Geometry check sheet. Reference: drawing and pictorial views, mm from the part's lowest x, y, z. A direction names the side the tool comes from. Round coordinates to 2 decimals unless told otherwise and drop trailing zeros. Put each result on its own line as item: value. Start each with the question number.
(1) Material ranges on probe 1 along X at (y, z) = (1.25, 42.5); probe 2 along X at (y, z) = (8.9, 42.5) (1 decimal); probe 3 along Y at (x, z) = (30.5, 8.5), recorded low to high.
(2) Section check B-B on y = 12. Count the separate pieces of the cut face and the enclosed holes in it.
(3) Gauge pin test, flat ends, axial feed: pin 1 (5 mm diameter, centred on y = 6, z = 53, fed in from -X); pin 2 (21 mm diameter, centred on x = 46.5, z = 56, fed in from -Y); pin 3 (10 mm diameter, centred on x = 14, y = 15.5, fed in from +Z) (1 decimal). Record the tip position at first contact, or that the pin passes through.
(4) Tool access check on the marked faces 1 and 2. Record the directions out of +Z, -Z, +X, -X, +Y, -Y that give a thin tool (end or side, any length) a straight path to the whole face; none if there is none.
(5) Mould release check, pull along X, two halves, no side actions. Record for the marked faces 3, 4, 5 and 6: pulls with the +X half, pulls with the -X half, needs draft (parallel to the pull), parting line crosses it, or undercut.
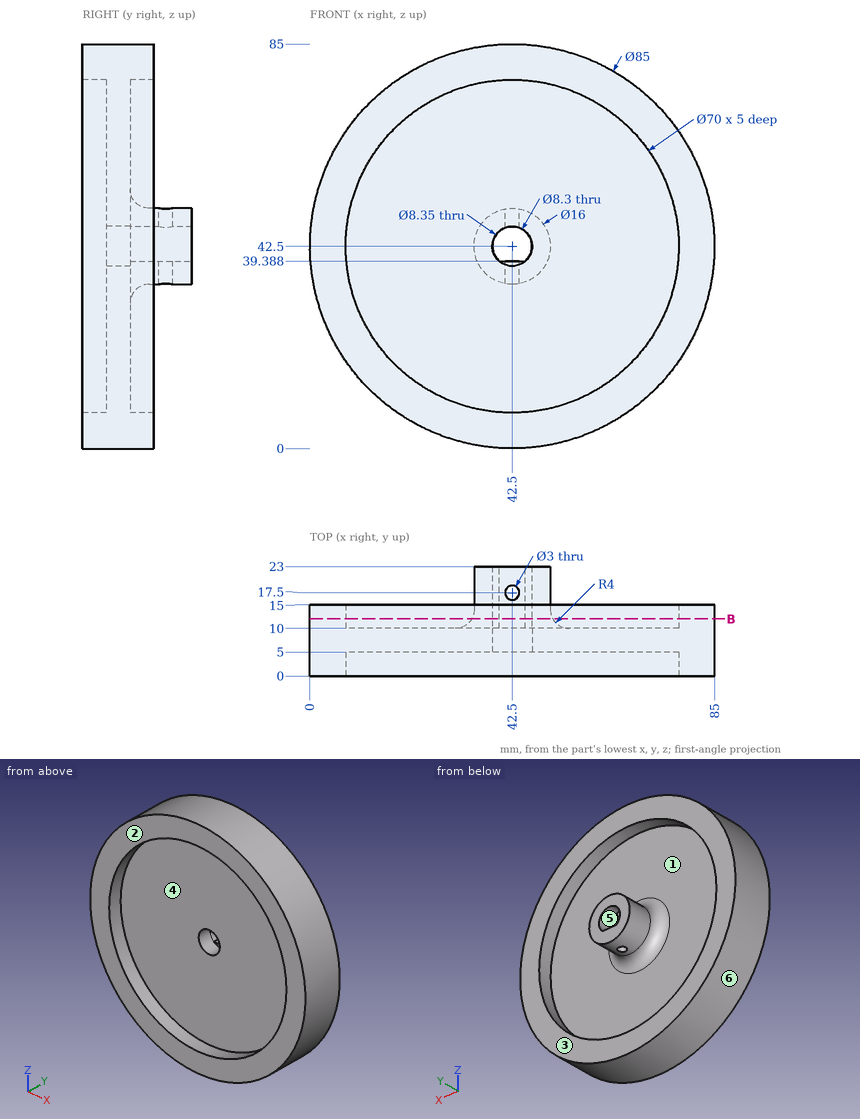
Answers follow:
1. probe 1: x = 0 to 7.5, 77.5 to 85
1. probe 2: x = 0 to 38.3, 46.7 to 85
1. probe 3: y = 0 to 15
2. separate pieces: 2
2. enclosed holes: 2
3. pin 1: stops at x = 0.76
3. pin 2: stops at y = 5
3. pin 3: stops at z = 77.9
4. face 1: +Y
4. face 2: +Z, -Z, +X, -X, -Y
5. face 3: needs draft
5. face 4: undercut
5. face 5: undercut
5. face 6: parting line crosses it
